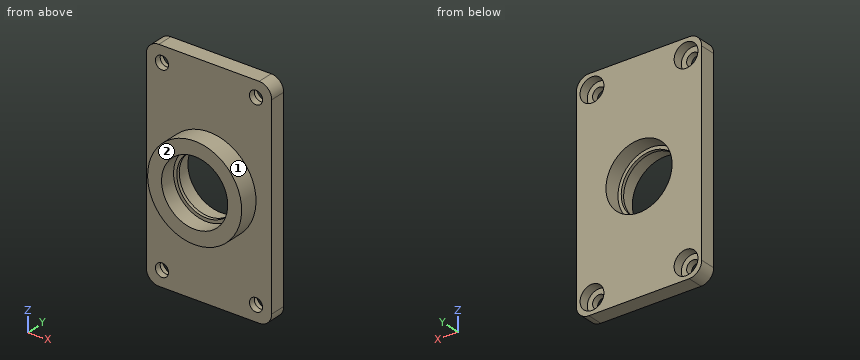
```python
from build123d import *

# Parameters (mm, degrees)
SKETCH_1_W          = 40
SKETCH_1_H          = 70
SKETCH_1_R          = 2.1
EXTRUDE_1_DEPTH     = 11
SKETCH_2_R          = 9.5
CUT_EXTRUDE_1_DEPTH = 11
SKETCH_3_R          = 10.55
CUT_EXTRUDE_2_DEPTH = 5
CUT_EXTRUDE_START   = -5
SKETCH_4_R          = 10.55
CUT_EXTRUDE_3_DEPTH = 5
SKETCH_5_W          = 40
SKETCH_5_H          = 70
SKETCH_5_R          = 15
CUT_EXTRUDE_4_DEPTH = 6
SKETCH_6_R          = 3.8
CUT_EXTRUDE_5_DEPTH = 3
FILLET_1_R          = 4


with BuildPart() as part:
    # 草图1 → 凸台-拉伸1 (new body)
    with BuildSketch(Plane(origin=(0, 0, 0), x_dir=(1, 0, 0), z_dir=(0, 1, 0))):
        Rectangle(SKETCH_1_W, SKETCH_1_H)
        with Locations(Location((-15, -30, 0), (0, 0, 270))):
            Circle(SKETCH_1_R, mode=Mode.SUBTRACT)
        with Locations(Location((15, -30, 0), (0, 0, 90))):
            Circle(SKETCH_1_R, mode=Mode.SUBTRACT)
        with Locations(Location((15, 30, 0), (0, 0, 270))):
            Circle(SKETCH_1_R, mode=Mode.SUBTRACT)
        with Locations(Location((-15, 30, 0), (0, 0, 90))):
            Circle(SKETCH_1_R, mode=Mode.SUBTRACT)
    extrude(amount=EXTRUDE_1_DEPTH)

    # 草图2 → 切除-拉伸1 (cut)
    with BuildSketch(Plane(origin=(0, 11, 0), x_dir=(1, 0, 0), z_dir=(0, 1, 0))):
        with Locations(Location((0, 0, 0), (0, 0, 270))):
            Circle(SKETCH_2_R)
    extrude(amount=-CUT_EXTRUDE_1_DEPTH, mode=Mode.SUBTRACT)

    # 草图3 → 切除-拉伸2 (cut)
    with BuildSketch(Plane(origin=(0, 11, 0), x_dir=(1, 0, 0), z_dir=(0, 1, 0))):
        with Locations(Location((0, 0, 0), (0, 0, 270))):
            Circle(SKETCH_3_R)
    extrude(amount=-CUT_EXTRUDE_2_DEPTH, mode=Mode.SUBTRACT)

    # 草图4 → 切除-拉伸3 (cut)
    with BuildSketch(Plane.XZ.offset(CUT_EXTRUDE_START)):
        with Locations(Location((0, 0, 0), (0, 0, 90))):
            Circle(SKETCH_4_R)
    extrude(amount=CUT_EXTRUDE_3_DEPTH, mode=Mode.SUBTRACT)

    # 草图5 → 切除-拉伸4 (cut)
    with BuildSketch(Plane.XZ):
        Rectangle(SKETCH_5_W, SKETCH_5_H)
        with Locations(Location((0, 0, 0), (0, 0, 270))):
            Circle(SKETCH_5_R, mode=Mode.SUBTRACT)
    extrude(amount=-CUT_EXTRUDE_4_DEPTH, mode=Mode.SUBTRACT)

    # 草图6 → 切除-拉伸5 (cut)
    with BuildSketch(Plane(origin=(0, 11, 0), x_dir=(1, 0, 0), z_dir=(0, 1, 0))):
        with Locations(Location((-15, 30, 0), (0, 0, 270))):
            Circle(SKETCH_6_R)
        with Locations(Location((15, 30, 0), (0, 0, 270))):
            Circle(SKETCH_6_R)
        with Locations(Location((15, -30, 0), (0, 0, 90))):
            Circle(SKETCH_6_R)
        with Locations(Location((-15, -30, 0), (0, 0, 90))):
            Circle(SKETCH_6_R)
    extrude(amount=-CUT_EXTRUDE_5_DEPTH, mode=Mode.SUBTRACT)

    # 圆角1
    fillet_1_edges = [part.edges().sort_by_distance(p)[0] for p in [
        (20, 8.5, 35),
        (-20, 8.5, 35),
        (-20, 8.5, -35),
        (20, 8.5, -35),
    ]]
    fillet(fillet_1_edges, radius=FILLET_1_R)


solid = part.part
```
Read the model definition and answer for the solid it produces. Units are mm, in the model's axes. Face numbers are marked on the shaded views. A direction names the side the tool comes from. Give positions to 0.01 mm unless a question says otherwise; leave off trailing zeros. Order: outer loops, then holes, each group sorted by start corner. A loop starts at its lowest first (then second) coordinate and runs counter-clockwise, first axis right, second up.
(1) Straight lines are drawn through the part: L1, parallel to X at y = 8.8, z = 30; L2, parallel to X at y = 7, z = 30; L3, parallel to X at y = 5.3, z = 0. For each, find the intervals that lie inside material, in ascending order.
(2) Find section C-C (x = 0). Give the vertices of the cut face in (y, z).
(3) Find section A-A (z = 30). Give the vertices of the cut face in (x, y), plus the area to 3 significant figures.
(4) For the marked faces 1 and 2, determine the directions among +Z, -Z, +X, -X, +Y, -Y from which every point of the face is accessible in a straight line to the end or side of a thin tool.
(5) Find section D-D (z = 0). Give the vertices of the cut face in (x, y).
(6) Given pin 1 (5 mm diameter, centred on x = -15, z = 30, fed in from -Y); pin 2 (4 mm diameter, centred on x = 15.5, z = -29.5, fed in from +Y); pin 3 (4 mm diameter, centred on x = 14, y = 3, fed in from +Z), each flat-ended and moving along its own axis, determine where each tip first touches the part or whether it passes through.
(7) Find section B-B (y = 9.5). Give the vertices of the cut face in (x, z), plus the area to 3 significant figures.
Result sheet:
1. L1: x = -20 to -18.8, -11.2 to 11.2, 18.8 to 20
1. L2: x = -20 to -17.1, -12.9 to 12.9, 17.1 to 20
1. L3: x = -15 to -9.5, 9.5 to 15
2. outline: (0, -15) - (6, -15) - (6, -35) - (11, -35) - (11, -10.55) - (6, -10.55) - (6, -9.5) - (5, -9.5) - (5, -10.55) - (0, -10.55) - close; (0, 10.55) - (5, 10.55) - (5, 9.5) - (6, 9.5) - (6, 10.55) - (11, 10.55) - (11, 35) - (6, 35) - (6, 15) - (0, 15) - close
3. outline: (-20, 6) - (-17.1, 6) - (-17.1, 8) - (-18.8, 8) - (-18.8, 11) - (-20, 11) - close; (-12.9, 6) - (12.9, 6) - (12.9, 8) - (11.2, 8) - (11.2, 11) - (-11.2, 11) - (-11.2, 8) - (-12.9, 8) - close; (17.1, 6) - (20, 6) - (20, 11) - (18.8, 11) - (18.8, 8) - (17.1, 8) - close
3. area: 138 mm2
4. face 1: -Y
4. face 2: +Z, -Z, +X, -X, -Y
5. outline: (-20, 6) - (-15, 6) - (-15, 0) - (-10.55, 0) - (-10.55, 5) - (-9.5, 5) - (-9.5, 6) - (-10.55, 6) - (-10.55, 11) - (-20, 11) - close; (9.5, 5) - (10.55, 5) - (10.55, 0) - (15, 0) - (15, 6) - (20, 6) - (20, 11) - (10.55, 11) - (10.55, 6) - (9.5, 6) - close
6. pin 1: stops at y = 6
6. pin 2: stops at y = 8
6. pin 3: stops at z = 9
7. outline: (-20, -31) arc R4 ccw to (-16, -35) - (16, -35) arc R4 ccw to (20, -31) - (20, 31) arc R4 ccw to (16, 35) - (-16, 35) arc R4 ccw to (-20, 31) - close; hole circle Ø7.6 at (-15, -30); hole circle Ø7.6 at (-15, 30); hole circle Ø21.1 at (0, 0); hole circle Ø7.6 at (15, -30); hole circle Ø7.6 at (15, 30)
7. area: 2,260 mm2
